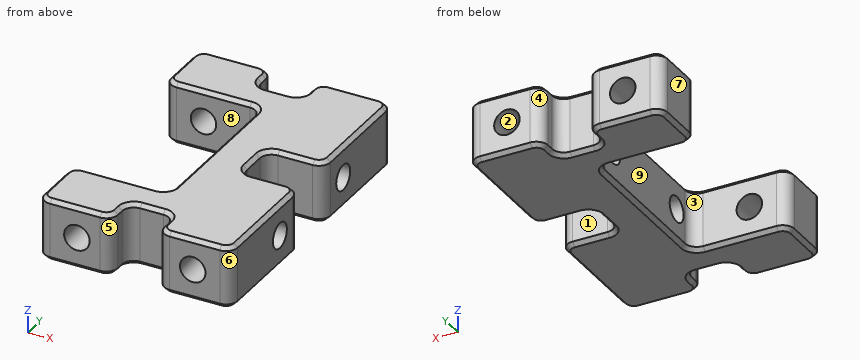
from build123d import *

# Parameters (mm, degrees)
EXTRUDE_1_DEPTH             = 4
SKETCH_2_R                  = 1.5
CUT_EXTRUDE_1_DEPTH         = 8
SKETCH_3_R                  = 1.5
CUT_EXTRUDE_2_DEPTH         = 24.092206478
HOLE_WIZARD_M4_1_D          = 3.3
HOLE_WIZARD_M4_2_AT_2_COUNT = 2
HOLE_WIZARD_M4_2_AT_2_PITCH = 15
SKETCH_9_W                  = 15
SKETCH_9_H                  = 6
SKETCH_9_W_2                = 6
SKETCH_9_H_2                = 8
CUT_EXTRUDE_3_DEPTH         = 25.109126902
FILLET_1_R                  = 1.5
CHAMFER_1_SIZE              = 0.5


with BuildPart() as part:
    # 草图1 → 凸台-拉伸1 (new, symmetric)
    with BuildSketch(Plane.XY):
        Polygon((12.5, 19), (-12.5, 19), (-12.5, 11), (0, 11), (0, -11), (-12.5, -11), (-12.5, -19), (12.5, -19), align=None)
    extrude(amount=EXTRUDE_1_DEPTH, both=True)

    # 草图2 → 切除-拉伸1 (cut)
    with BuildSketch(Plane(origin=(0, 19, 0), x_dir=(1, 0, 0), z_dir=(0, 1, 0))):
        with Locations(Location((-7.5, 0, 0), (0, 0, 270))):
            Circle(SKETCH_2_R)
        with Locations(Location((7.5, 0, 0), (0, 0, 270))):
            Circle(SKETCH_2_R)
    extrude(amount=-CUT_EXTRUDE_1_DEPTH, mode=Mode.SUBTRACT)

    # 草图3 → 切除-拉伸2 (cut, through all)
    with BuildSketch(Plane.ZY):
        with Locations((0, 7.5)):
            Circle(SKETCH_3_R)
        with Locations((0, -7.5)):
            Circle(SKETCH_3_R)
    extrude(amount=-CUT_EXTRUDE_2_DEPTH, mode=Mode.SUBTRACT)

    # M4 螺纹孔1 (through all)
    with Locations(Plane(origin=(12.5, 0, 0), x_dir=(0, 0, -1), z_dir=(1, 0, 0))):
        with Locations((0, 7.5), (0, -7.5)):
            Hole(HOLE_WIZARD_M4_1_D / 2)

    # 草图8 → M4 螺纹孔2 (revolve, cut)
    with BuildSketch(Plane(origin=(-7.5, 19, 0), x_dir=(0, 0, 1), z_dir=(1, 0, 0))):
        Polygon((0, 0), (0, 8.991420021), (1.65, 8), (1.65, 0), align=None)
    hole_wizard_m4_2 = revolve(axis=Axis((-7.5, 25.35, 0), (0, -1, 0)), mode=Mode.SUBTRACT)

    # M4 螺纹孔2 at 2: M4 螺纹孔2 ×2
    with Locations(*[(i * HOLE_WIZARD_M4_2_AT_2_PITCH, 0, 0) for i in range(1, HOLE_WIZARD_M4_2_AT_2_COUNT)]):
        add(hole_wizard_m4_2, mode=Mode.SUBTRACT)

    # 镜向1: M4 螺纹孔2 across plane
    add(hole_wizard_m4_2.mirror(Plane.ZX), mode=Mode.SUBTRACT)

    # 镜向1 copy 1 sketch → 镜向1 copy 1 (revolve, cut)
    with BuildSketch(Plane(origin=(7.5, -19, 0), x_dir=(0, 0, 1), z_dir=(1, 0, 0))):
        Polygon((0, 0), (0, -8.991420021), (1.65, -8), (1.65, 0), align=None)
    revolve(axis=Axis((7.5, -25.35, 0), (0, -1, 0)), mode=Mode.SUBTRACT)

    # 草图9 → 切除-拉伸3 (cut, through all)
    with BuildSketch(Plane.XY.offset(4)):
        with Locations((12.5, 0)):
            Rectangle(SKETCH_9_W, SKETCH_9_H)
        with Locations((0, 19)):
            Rectangle(SKETCH_9_W_2, SKETCH_9_H_2)
        with Locations((0, -19)):
            Rectangle(SKETCH_9_W_2, SKETCH_9_H_2)
    extrude(amount=-CUT_EXTRUDE_3_DEPTH, mode=Mode.SUBTRACT)

    # 圆角1
    fillet_1_edges = [part.edges().sort_by_distance(p)[0] for p in [
        (3, 19, 0),
        (-3, 19, 0),
        (3, 15, 0),
        (-3, 15, 0),
        (3, -19, 0),
        (3, -15, 0),
        (-3, -19, 0),
        (-3, -15, 0),
        (-12.5, 11, 0),
        (-12.5, 19, 0),
        (12.5, 19, 0),
        (12.5, -19, 0),
        (-12.5, -19, 0),
        (-12.5, -11, 0),
        (0, -11, 0),
        (0, 11, 0),
        (12.5, 3, 0),
        (12.5, -3, 0),
        (5, -3, 0),
        (5, 3, 0),
    ]]
    fillet(fillet_1_edges, radius=FILLET_1_R)

    # 倒角1
    chamfer_1_edges = [part.edges().sort_by_distance(p)[0] for p in [
        (7.75, -19, 4),
        (7.75, -19, -4),
        (12.5, 11, -4),
        (8.75, 3, -4),
        (5, 0, -4),
        (8.75, -3, -4),
        (12.5, -11, -4),
        (3, -17, -4),
        (0, -15, -4),
        (-3, -17, -4),
        (-7.75, -19, -4),
        (-12.5, -15, -4),
        (-6.25, -11, -4),
        (0, 0, -4),
        (-6.25, 11, -4),
        (-12.5, 15, -4),
        (-7.75, 19, -4),
        (-3, 17, -4),
        (0, 15, -4),
        (3, 17, -4),
        (7.75, 19, -4),
        (-12.060660172, 11.439339828, -4),
        (-12.060660172, -11.439339828, -4),
        (-12.060660172, -18.560660172, -4),
        (12.060660172, -18.560660172, -4),
        (12.060660172, 18.560660172, -4),
        (-12.060660172, 18.560660172, -4),
        (12.060660172, -3.439339828, -4),
        (12.060660172, 3.439339828, -4),
        (3.439339828, 18.560660172, -4),
        (-3.439339828, 18.560660172, -4),
        (-3.439339828, -18.560660172, -4),
        (3.439339828, -18.560660172, -4),
        (3, -17, 4),
        (8.75, 3, 4),
        (12.5, 11, 4),
        (7.75, 19, 4),
        (3, 17, 4),
        (0, 15, 4),
        (-3, 17, 4),
        (-7.75, 19, 4),
        (-12.5, 15, 4),
        (-6.25, 11, 4),
        (0, 0, 4),
        (-6.25, -11, 4),
        (-12.5, -15, 4),
        (-7.75, -19, 4),
        (-3, -17, 4),
        (0, -15, 4),
        (12.5, -11, 4),
        (8.75, -3, 4),
        (5, 0, 4),
        (-12.060660172, 11.439339828, 4),
        (-12.060660172, -11.439339828, 4),
        (-12.060660172, -18.560660172, 4),
        (12.060660172, -18.560660172, 4),
        (12.060660172, 18.560660172, 4),
        (-12.060660172, 18.560660172, 4),
        (12.060660172, -3.439339828, 4),
        (12.060660172, 3.439339828, 4),
        (3.439339828, 18.560660172, 4),
        (-3.439339828, 18.560660172, 4),
        (-3.439339828, -18.560660172, 4),
        (3.439339828, -18.560660172, 4),
        (2.560660172, -15.439339828, 4),
        (2.560660172, -15.439339828, -4),
        (-2.560660172, -15.439339828, 4),
        (-2.560660172, -15.439339828, -4),
        (-2.560660172, 15.439339828, 4),
        (-2.560660172, 15.439339828, -4),
        (2.560660172, 15.439339828, 4),
        (2.560660172, 15.439339828, -4),
        (5.439339828, 2.560660172, 4),
        (5.439339828, 2.560660172, -4),
        (5.439339828, -2.560660172, 4),
        (5.439339828, -2.560660172, -4),
        (-0.439339828, -10.560660172, -4),
        (-0.439339828, -10.560660172, 4),
        (-0.439339828, 10.560660172, -4),
        (-0.439339828, 10.560660172, 4),
    ]]
    chamfer(chamfer_1_edges, length=CHAMFER_1_SIZE)


solid = part.part
Build history of the part. All positions in model axes, mm. Face numbers are marked on the shaded views. A direction names the side the tool comes from. Give positions to 0.01 mm unless a question says otherwise; leave off trailing zeros. Order: outer loops, then holes, each group sorted by start corner. A loop starts at its lowest first (then second) coordinate and runs counter-clockwise, first axis right, second up. Notation, with made-up numbers: M 22.5,27.5 L 62.5,27.5 A27 cw 62.5,51.5 Z; hole C 6.25,75.25 d1. An arc over 180 degrees is marked long. Use one line per item in the form item = value.
Q1. Slice it at A-A, the plane x = -7.5. Write the cut outline in (y, z).
Conclusion:
outline = M -19,-3.5 L -18.5,-4 L -11.5,-4 L -11,-3.5 L -11,-1.65 L -19,-1.65 Z; M -19,1.65 L -11,1.65 L -11,3.5 L -11.5,4 L -18.5,4 L -19,3.5 Z; M 11,-3.5 L 11.5,-4 L 18.5,-4 L 19,-3.5 L 19,-1.65 L 11,-1.65 Z; M 11,1.65 L 19,1.65 L 19,3.5 L 18.5,4 L 11.5,4 L 11,3.5 Z
Q2. Wall check: probe 1 along X at (y, z) = (-14, 0); probe 2 along Y at (x, z) = (9.5, 0); probe 3 along Z at (x, y) = (-7.5, -15.5). Give the ranges that are in metal, low to high.
Conclusion:
probe_1 = -12.5 to -9.15, -5.85 to 5.85, 9.15 to 12.5
probe_2 = -19 to -9.15, -5.85 to -3, 3 to 5.85, 9.15 to 19
probe_3 = -4 to -1.65, 1.65 to 4
Q3. Which spindle directions (+Z, -Z, +X, -X, +Y, -Y) get a long thin tool onto all of the face, cutting with end or side? Do the marked faces 1, 2, 3, 4 and 5. Say none if no direction does.
Conclusion:
face_1 = +Z, -Z, +X
face_2 = +Y
face_3 = +Z, -Z, -X
face_4 = +Z, -Z, +Y
face_5 = +Z, -Z, -Y
Q4. Pull direction Y, two halves, no side cores. Call the marked faces 6, 7, 8 and 9: released by +Y, released by -Y, zero draft, split by the parting line, or undercut.
Conclusion:
face_6 = released by -Y
face_7 = zero draft
face_8 = undercut
face_9 = undercut
Q5. Pin check, flat tips, straight feed: P1, Ø1.5, axis at x = -0.5, z = 0.5, coming from the -Y side; P2, Ø1.5, axis at y = -0.5, z = 0.5, coming from the +X side; P3, Ø1.5, axis at x = 0, z = 1.5, coming from the +Y side. Stop position of each tip, or through.
Conclusion:
P1 = -15
P2 = 5
P3 = 15
Q6. Slice it at B-B, the plane y = -7.5. Write the cut outline in (x, z), and give its area (4 significant figures).
Conclusion:
outline = M 0,-3.5 L 0.5,-4 L 12,-4 L 12.5,-3.5 L 12.5,-1.65 L 0,-1.65 Z; M 0,1.65 L 12.5,1.65 L 12.5,3.5 L 12,4 L 0.5,4 L 0,3.5 Z
area = 58.25 mm2
Q7. Slice it at C-C, the plane y = 0.5. Write the cut outline in (x, z), and give its area (3 significant figures).
Conclusion:
outline = M 0,-3.5 L 0.5,-4 L 4.5,-4 L 5,-3.5 L 5,3.5 L 4.5,4 L 0.5,4 L 0,3.5 Z
area = 39.5 mm2
Q8. Slice it at D-D, the plane z = 1.25. State how many separate pieces and enclosed holes the cut face has, and give its area (3 significant figures).
Conclusion:
separate_pieces = 5
enclosed_holes = 0
area = 457 mm2
